Answer from the drawing. Dimensions are ordinates in mm from the lowest x, y and z of the part. A direction names the side the tool comes from. Give positions to 0.01 mm unless a question says otherwise; leave off trailing zeros. Write each loop counter-clockwise with the first axis right and the second up, starting at its lowest first coordinate (ties: lowest second). Pieces come first, ordered by that corner, then holes.
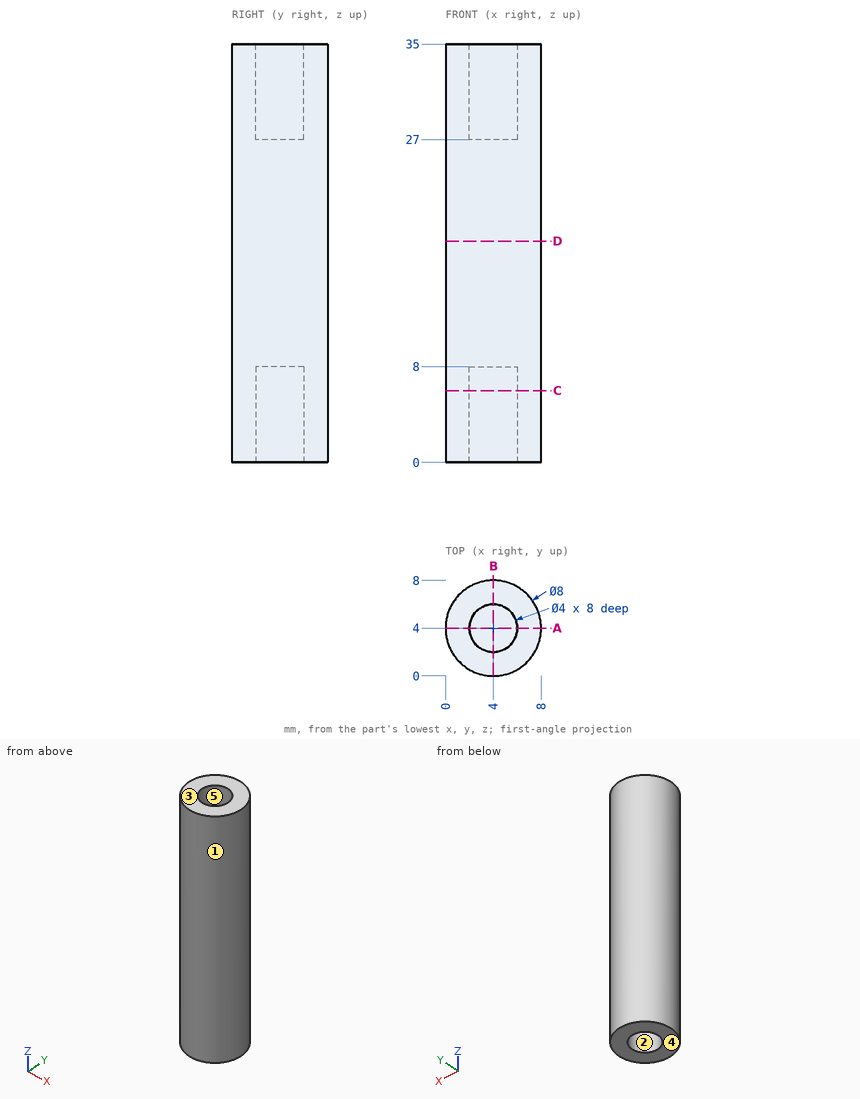
Item 1: Find the intervals of material crossed by line 1 along Y through (x, z) = (4, 5.5); line 2 along Z through (x, y) = (3.5, 5.25); line 3 along Y through (x, z) = (3.75, 26.5), in increasing order.
Result set:
line 1: y = 0 to 2, 6 to 8
line 2: z = 8 to 27
line 3: y = 0.01 to 7.99
Item 2: Section D-D (z = 18.5) is taken. Write down the section's boundary in (x, y).
Result set:
outline: circle Ø8 at (4, 4)
Item 3: Which of the six approach directions +Z, -Z, +X, -X, +Y, -Y give full straight-line access (tool end or side, diameter ignored) to the marked faces 4 and 5?
Result set:
face 4: -Z, +X, -X, +Y, -Y
face 5: +Z
Item 4: Section A-A (y = 4) is taken. Write down the section's boundary in (x, z).
Result set:
outline: (0, 0) - (2, 0) - (2, 8) - (6, 8) - (6, 0) - (8, 0) - (8, 35) - (6, 35) - (6, 27) - (2, 27) - (2, 35) - (0, 35) - close
Item 5: Section C-C (z = 6) is taken. Write down the section's boundary in (x, y).
Result set:
outline: circle Ø8 at (4, 4); hole circle Ø4 at (4, 4)
Item 6: Determine the mould class of the marked faces 1, 2 and 3 for opening direction Y: pulls with the +Y half, pulls with the -Y half, needs draft (parallel to the pull), parting line crosses it, or undercut.
Result set:
face 1: parting line crosses it
face 2: undercut
face 3: needs draft
Item 7: Each of these flat-tipped pins is pushed along its axis until it touches: pin 1 Ø2 at (x, y) = (4.5, 4) entering from +Z; pin 2 Ø2 at (x, y) = (3.5, 3.5) entering from -Z. Where does it stop, or does it pass through?
Result set:
pin 1: stops at z = 27
pin 2: stops at z = 8
